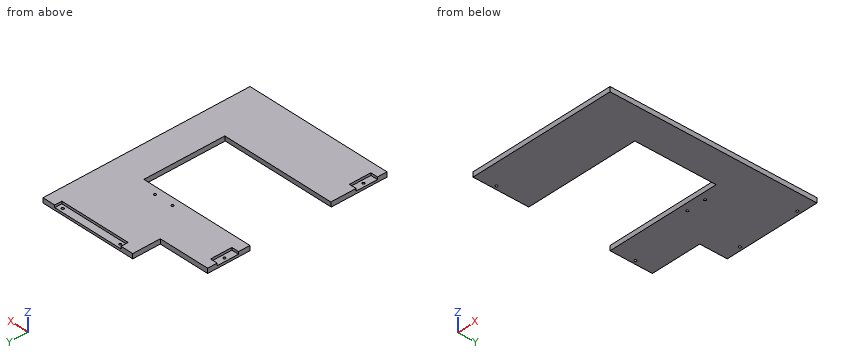
Autodesk Inventor part; units mm, degrees
ref_plane "YZ Plane" through (0, 0, 0) normal (1, 0, 0) x (0, 1, 0)
ref_plane "XZ Plane" through (0, 0, 0) normal (0, 1, 0) x (-1, 0, 0)
ref_plane "XY Plane" through (0, 0, 0) normal (0, 0, 1) x (1, 0, 0)
sketch "Sketch1" plane through (0, 0, 0) normal (0, 0, 1) x (1, 0, 0)
  line L0 (0, 0) -> (620, 0)
  line L1 (620, 0) -> (620, 620)
  line L2 (620, 620) -> (0, 620)
  line L3 (0, 620) -> (0, 0)
  line L4 (203, 491) -> (417, 491)
  line L5 (417, 491) -> (417, 377)
  line L6 (417, 377) -> (203, 377)
  line L7 (203, 377) -> (203, 491)
  line L8 (620, 0) -> (310, 0)
  line L9 (310, 0) -> (310, 435)
  line L10 (310, 435) -> (620, 435)
  line L11 (620, 435) -> (620, 0)
  point P0 (310, 491)
  point P1 (310, 620)
  dimension "d0" = 620
  dimension "d1" = 620
  dimension "d2" = 214
  dimension "d3" = 114
  dimension "d4" = 129
  dimension "d28" = 435
extrude "Extrusion1" add sketch "Sketch1" along normal blind 10 contours L3 L2 L1 L10 L5 L4 L7 L6 L9 L0 | L9 L6 L5 L10 L1 L0
sketch "Sketch6" plane through (0, 0, 10) normal (0, 0, 1) x (1, 0, 0)
  line L0 (0, 0) -> (620, 0)
  line L1 (620, 0) -> (310, 0)
  line L2 (310, 0) -> (310, 435)
  line L3 (310, 435) -> (620, 435)
  line L4 (620, 435) -> (620, 0)
  line L5 (620, 620) -> (0, 620)
  line L6 (620, 435) -> (0, 435)
  line L7 (0, 435) -> (0, 620)
  line L8 (0, 620) -> (620, 620)
  line L9 (620, 620) -> (620, 435)
  line L10 (310, 435) -> (0, 435)
  line L11 (0, 435) -> (0, 0)
  line L12 (0, 0) -> (310, 0)
  line L13 (310, 0) -> (310, 435)
  point P0 (310, 620)
  dimension "d29" = 435
extrude "Extrusion6" cut sketch "Sketch6" against normal through all contours L11 L6 L2 L0 | L7 L5 L9 L3 L6
sketch "Sketch7" plane through (0, 0, 10) normal (0, 0, 1) x (1, 0, 0)
  line L0 (310, 377) -> (310, 0)
  line L1 (417, 435) -> (620, 435)
  line L2 (443.5, 435) -> (593.5, 435)
  line L3 (593.5, 435) -> (593.5, 420)
  line L4 (593.5, 420) -> (443.5, 420)
  line L5 (443.5, 420) -> (443.5, 435)
  line L6 (310, 357) -> (325, 357)
  line L7 (325, 357) -> (325, 312)
  line L8 (325, 312) -> (310, 312)
  line L9 (310, 312) -> (310, 357)
  line L10 (310, 20) -> (325, 20)
  line L11 (325, 20) -> (325, 65)
  line L12 (325, 65) -> (310, 65)
  line L13 (310, 65) -> (310, 20)
  line L14 (417, 377) -> (310, 377)
  line L15 (310, 0) -> (620, 0)
  point P0 (0, 0)
  point P1 (518.5, 435)
  dimension "d34" = 150
  dimension "d35" = 15
  dimension "d48" = 15
  dimension "d49" = 45
  dimension "d50" = 15
  dimension "d51" = 45
  dimension "d52" = 20
  dimension "d53" = 20
extrude "Extrusion7" cut sketch "Sketch7" against normal blind 5
sketch "Sketch8" plane through (0, 0, 5) normal (0, 0, 1) x (1, 0, 0)
  circle A0 centre (453.5, 427.5) radius 2.5
  circle A1 centre (583.5, 427.5) radius 2.5
  circle A2 centre (317.5, 334.5) radius 2.5
  circle A3 centre (317.5, 42.5) radius 2.5
  line L0 (310, 312) -> (310, 357)
  line L1 (325, 312) -> (310, 312)
  line L2 (325, 357) -> (325, 312)
  line L3 (310, 357) -> (325, 357)
  line L4 (443.5, 420) -> (443.5, 435)
  line L5 (593.5, 420) -> (443.5, 420)
  line L6 (593.5, 435) -> (593.5, 420)
  line L7 (443.5, 435) -> (593.5, 435)
  line L8 (310, 20) -> (310, 65)
  line L9 (325, 20) -> (310, 20)
  line L10 (325, 65) -> (325, 20)
  line L11 (310, 65) -> (325, 65)
  line L12 (310, 20) -> (310, 65)
  point P0 (0, 0)
  point P1 (593.5, 427.5)
  point P2 (443.5, 427.5)
  point P3 (317.5, 357)
  point P4 (317.5, 65)
  point P5 (310, 42.5)
  point P6 (310, 334.5)
  dimension "d38" = 5
  dimension "d39" = 5
  dimension "d40" = 5
  dimension "d54" = 10
  dimension "d55" = 10
extrude "Extrusion8" cut sketch "Sketch8" against normal through all contours A0 | A1 | A2 | A3
sketch "Sketch9" plane through (0, 0, 10) normal (0, 0, 1) x (1, 0, 0)
  line L0 (550, 288) -> (310, 288)
  line L1 (310, 288) -> (310, 118)
  line L2 (310, 118) -> (550, 118)
  line L3 (550, 118) -> (550, 288)
  line L4 (310, 312) -> (310, 65)
  line L5 (325, 312) -> (310, 312)
  point P0 (0, 0)
  dimension "d56" = 240
  dimension "d57" = 170
  dimension "d67" = 24
extrude "Extrusion9" cut sketch "Sketch9" against normal through all
sketch "Sketch10" plane through (0, 0, 10) normal (0, 0, 1) x (1, 0, 0)
  circle A0 centre (509, 303) radius 2.5
  circle A1 centre (469, 303) radius 2.5
  line L0 (550, 288) -> (550, 118)
  line L1 (310, 288) -> (550, 288)
  point P0 (0, 0)
  dimension "d60" = 5
  dimension "d61" = 5
  dimension "d62" = 41
  dimension "d63" = 40
  dimension "d64" = 15
extrude "Extrusion10" cut sketch "Sketch10" along normal through all both and the other way through all
chamfer "Chamfer1" distance 10 angle 5 1 edges at (430, 118, 0) measured on face at (390, 118, 6.6667)
properties part number "TC001b" material "ABS Plastic"
The model under review builds one solid part; all positions refer to its coordinate system, in mm. Round coordinates to 2 decimals unless told otherwise and drop trailing zeros. Order: outer loops, then holes, each group sorted by start corner. A loop starts at its lowest first (then second) coordinate and runs counter-clockwise, first axis right, second up. Notation, with made-up numbers: (36.5, -21.75) -> (82.5, -21.75) arc R21 ccw to (82.5, 13.25) -> close; hole circle Ø11 at (55, -9.75). An arc over 180 degrees is marked (long way). Use a Markdown table: item, result.
Q1. Clearance check with flat-ended pins moving along their axes: P1, Ø5, axis at y = 412, z = 4.5, coming from the -X side; P2, Ø3, axis at x = 317.5, y = 334.5, coming from the +Z side; P3, Ø5.5, axis at x = 317, z = 8, coming from the -Y side; P4, Ø1.5, axis at x = 317.5, z = 8.5, coming from the +Y side. State where each tip first meets the part, or that it passes through.
Values:
| item | result |
|---|---|
| P1 | stops at x = 417 |
| P2 | passes through |
| P3 | stops at y = 0 |
| P4 | stops at y = 377 |
Q2. For line 1 (X direction, y = 427.5, z = 2.4); line 2 (X direction, y = 303, z = 5.25); line 3 (Y direction, x = 481.5, z = 0.75), list the stretches that pass through material, from the lowest coordinate up.
Values:
| item | result |
|---|---|
| line 1 | x = 417 to 451, 456 to 581, 586 to 620 |
| line 2 | x = 310 to 466.5, 471.5 to 506.5, 511.5 to 620 |
| line 3 | y = 0 to 117.19, 288 to 435 |
Q3. We need section D-D on y = 238. Write out the cut boundary in (x, z), then the cut area to 3 significant figures.
Values:
| item | result |
|---|---|
| outline | (550, 0) -> (620, 0) -> (620, 10) -> (550, 10) -> close |
| area | 700 mm^2 |
Q4. We need section B-B on z = 2.25. Write out the cut boundary in (x, y).
Values:
| item | result |
|---|---|
| outline | (310, 0) -> (620, 0) -> (620, 435) -> (417, 435) -> (417, 377) -> (310, 377) -> (310, 288) -> (550, 288) -> (550, 117.32) -> (310, 117.32) -> close; hole circle Ø5 at (317.5, 42.5); hole circle Ø5 at (317.5, 334.5); hole circle Ø5 at (453.5, 427.5); hole circle Ø5 at (469, 303); hole circle Ø5 at (509, 303); hole circle Ø5 at (583.5, 427.5) |
